from build123d import *

# Parameters (mm, degrees)
DODANIE_WYCI_GNI_CIE1_DEPTH      = 5
DODANIE_WYCI_GNI_CIE1_DEPTH_BACK = 28
SZKIC1_R                         = 2.4
SZKIC2_R                         = 4.5
DODANIE_WYCI_GNI_CIE2_DEPTH      = 4
SFAZOWANIE1_SIZE                 = 2
WYTNIJ_WYCI_GNI_CIE1_DEPTH       = 29.714108031
WYTNIJ_WYCI_GNI_CIE1_DEPTH_BACK  = 29.714108031
SZKIC3_R                         = 1


with BuildPart() as part:
    # Szkic1 → Dodanie-wyciągnięcie1 (new, two sides: drawn at the far end of the back side and taken through both)
    with BuildSketch(Plane(origin=(0, 0, 0), x_dir=(0, 0, -1), z_dir=(1, 0, 0)).offset(-DODANIE_WYCI_GNI_CIE1_DEPTH_BACK)):
        Circle(SZKIC1_R)
    extrude(amount=DODANIE_WYCI_GNI_CIE1_DEPTH + DODANIE_WYCI_GNI_CIE1_DEPTH_BACK)

    # Szkic2 → Dodanie-wyciągnięcie2 (add)
    with BuildSketch(Plane(origin=(5, 0, 0), x_dir=(0, 0, -1), z_dir=(1, 0, 0))):
        Circle(SZKIC2_R)
    extrude(amount=DODANIE_WYCI_GNI_CIE2_DEPTH)

    # Sfazowanie1
    sfazowanie1_edges = [part.edges().sort_by_distance(p)[0] for p in [
        (9, 0, 4.5),
    ]]
    chamfer(sfazowanie1_edges, length=SFAZOWANIE1_SIZE)

    # Szkic3 → Wytnij-wyciągnięcie1 (cut, two sides: drawn at the far end of the back side and taken through both)
    with BuildSketch(Plane(origin=(0, 0, 0), x_dir=(1, 0, 0), z_dir=(0, 1, 0)).offset(-WYTNIJ_WYCI_GNI_CIE1_DEPTH_BACK)):
        with Locations(Location((-26, 0, 0), (0, 0, 270))):
            Circle(SZKIC3_R)
    extrude(amount=WYTNIJ_WYCI_GNI_CIE1_DEPTH + WYTNIJ_WYCI_GNI_CIE1_DEPTH_BACK, mode=Mode.SUBTRACT)


solid = part.part
Source: CAD feature listing. Evaluate the final solid. Frame: model axes, mm. A direction names the side the tool comes from. Round coordinates to 2 decimals unless told otherwise and drop trailing zeros. Loops run counter-clockwise (first coordinate to the right, second up) from the corner with the lowest first, then second, coordinate; pieces in that order, holes last. Notation, with made-up numbers: (62.5, -15.75) -> (82.5, -15.75) arc R18 cw to (82.5, 17.25) -> close; hole circle Ø2 at (20.25, 76.25). An arc over 180 degrees is marked (long way). Answer as a JSON object with one key per item and string values. Group by question number.
Q1. Section query C-C (x = -26). Output: boundary loops of the cut face in (y, z), plus the area to 3 significant figures.
Q2. Mould query, pull axis X, two halves, no side actions, for faces 1 (the flat face through (5, -2, -2)), 2 (the flat face through (9, 0, 0)), 3 (the cylindrical face through (-27, 0, 0)). Classes: pulls with the +X half, pulls with the -X half, needs draft (parallel to the pull), parting line crosses it, or undercut.
Q3. Section query A-A (y = 0). Output: boundary loops of the cut face in (x, z), plus the area to 3 significant figures.
Q4. Section query B-B (x = -12). Output: boundary loops of the cut face in (y, z), plus the area to 3 significant figures.
Q5. Access query for faces 4 (the cylindrical face through (5.99, 4.46, 0.59)), 5 (the cylindrical face through (-11.73, 0.72, -2.29)). Directions: +Z, -Z, +X, -X, +Y, -Y. A direction counts if a zero-diameter tool reaches every point of the face in a straight line with its end or side. Return the directions, or none.
Q6. Ray query, line 1 (X direction, y = 0.5, z = 0); line 2 (Z direction, x = -26, y = 0.1); line 3 (Y direction, x = 0.5, z = 0). Return the intervals inside material, ascending. Write a range as from..to.
Q7. Contact query for flat-ended pins moving along their axis: P1, Ø2, axis at x = -2, z = -0.5, coming from the -Y side; P2, Ø5, axis at x = -5.5, y = 0.5, coming from the +Z side; P3, Ø2, axis at x = -6.5, y = 3, coming from the -Z side. Output: stop coordinate, or through.
Completed:
{
 "1": {"outline": "(-2.18, -1) arc R2.4 ccw to (2.18, -1) -> close; (-2.18, 1) -> (2.18, 1) arc R2.4 ccw to start", "area": "8.78 mm²"},
 "2": {"face 1": "pulls with the -X half", "face 2": "pulls with the +X half", "face 3": "undercut"},
 "3": {"outline": "(-28, -2.4) -> (5, -2.4) -> (5, -4.5) -> (7, -4.5) -> (9, -2.5) -> (9, 2.5) -> (7, 4.5) -> (5, 4.5) -> (5, 2.4) -> (-28, 2.4) -> close; hole circle Ø2 at (-26, 0)", "area": "187 mm²"},
 "4": {"outline": "circle Ø4.8 at (0, 0)", "area": "18.1 mm²"},
 "5": {"face 4": "+X, -X", "face 5": "-X"},
 "6": {"line 1": "-28..-27, -25..9", "line 2": "-2.4..-1, 1..2.4", "line 3": "-2.4..2.4"},
 "7": {"P1": "y = -2.4", "P2": "z = 2.4", "P3": "z = -1.33"}
}
